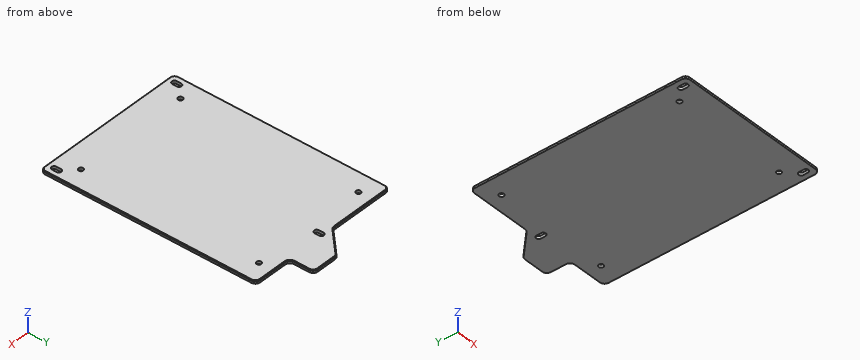
Autodesk Inventor part; units mm, degrees
ref_plane "YZ Plane" through (0, 0, 0) normal (1, 0, 0) x (0, 1, 0)
ref_plane "XZ Plane" through (0, 0, 0) normal (0, 1, 0) x (-1, 0, 0)
ref_plane "XY Plane" through (0, 0, 0) normal (0, 0, 1) x (1, 0, 0)
sketch "Sketch1" plane through (0, 0, 0) normal (0, 0, 1) x (1, 0, 0)
  line L0 (-82.5, -114.5) -> (82.5, -114.5)
  line L1 (82.5, -114.5) -> (82.5, 114.5)
  line L2 (82.5, 114.5) -> (-82.5, 114.5)
  line L3 (-82.5, 114.5) -> (-82.5, -114.5)
  line L4 (-82.5, -114.5) -> (82.5, 114.5) construction
  line L5 (82.5, -114.5) -> (-82.5, 114.5) construction
  circle A0 centre (61.5, 99.5) radius 2.5
  line L6 (-147.2223, 0) -> (154.3177, 0) construction
  line L7 (-104.1452, 5) -> (111.2405, 5) construction
  circle A1 centre (61.5, -89.5) radius 2.5
  line L8 (0, 191.5) -> (0, -165.5) construction
  circle A2 centre (-61.5, 99.5) radius 2.5
  circle A3 centre (-61.5, -89.5) radius 2.5
  line L9 (41.5, 114.5) -> (41.5, 140.5)
  line L10 (41.5, 140.5) -> (13.216, 140.5)
  line L11 (13.216, 140.5) -> (-12.784, 114.5)
  point P0 (0, 0)
  dimension "d0" = 229
  dimension "d1" = 165
  dimension "d3" = 5
  dimension "d5" = 189
  dimension "d6" = 25
  dimension "d9" = 61.5
  dimension "d31" = 41
  dimension "d32" = 26
  dimension "d33" = 135
  dimension "d34" = 28.284
extrude "Plate1" add sketch "Sketch1" along normal blind 3
fillet "Fillet1" radius 5 4 edges at (-82.5, 114.5, 1.5) (82.5, 114.5, 1.5) (82.5, -114.5, 1.5) (-82.5, -114.5, 1.5)
sketch "Sketch2" plane through (0, 0, 3) normal (0, 0, 1) x (1, 0, 0)
  line L0 (-74.3, -107) -> (-74.3, -102) construction
  line L1 (-76.95, -107) -> (-76.95, -102)
  line L2 (-71.65, -102) -> (-71.65, -107)
  arc A0 (-76.95, -107) -> (-71.65, -107) centre (-74.3, -107) ccw
  arc A1 (-71.65, -102) -> (-76.95, -102) centre (-74.3, -102) ccw
  line L3 (-103.0799, -19.5) -> (98.9164, -19.5) construction
  line L4 (0, 191.5) -> (0, -165.5) construction
  line L5 (-82.5, -109.5) -> (-82.5, 109.5) construction
  line L6 (74.3, -107) -> (74.3, -102) construction
  line L7 (76.95, -107) -> (76.95, -102)
  line L8 (71.65, -102) -> (71.65, -107)
  arc A2 (71.65, -107) -> (76.95, -107) centre (74.3, -107) ccw
  arc A3 (76.95, -102) -> (71.65, -102) centre (74.3, -102) ccw
  line L9 (77.5, -114.5) -> (-77.5, -114.5)
  line L10 (0, 113) -> (0, 108) construction
  line L11 (-2.65, 113) -> (-2.65, 108)
  line L12 (2.65, 108) -> (2.65, 113)
  arc A4 (2.65, 113) -> (-2.65, 113) centre (0, 113) ccw
  arc A5 (-2.65, 108) -> (2.65, 108) centre (0, 108) ccw
  line L13 (-77.5, 114.5) -> (77.5, 114.5)
  point P0 (0, 0)
  point P1 (-74.3, -104.5)
  point P2 (74.3, -104.5)
  point P3 (82.5, -109.5)
  point P4 (0, 110.5)
  dimension "d12" = 85
  dimension "d14" = 5
  dimension "d15" = 2.65
  dimension "d18" = 10
  dimension "d22" = 148.6
  dimension "d23" = 5
  dimension "d24" = 2.65
  dimension "d26" = 225
extrude "Cut1" cut sketch "Sketch2" against normal blind 3
fillet "Fillet2" radius 5 4 edges at (41.5, 114.5, 1.5) (41.5, 140.5, 1.5) (13.216, 140.5, 1.5) (-12.784, 114.5, 1.5)
chamfer "Chamfer1" distance 0.75 angle 45 14 edges at (0, -114.5, 3) (-81.0355, -113.0355, 3) (-82.5, 0, 3) (-81.0355, 113.0355, 3) (-46.1775, 114.5, 3) (13.3737, 140.1194, 3) (40.0355, 139.0355, 3) (0.216, 127.5, 3) (25.8935, 140.5, 3) (41.5, 127.5, 3) (62, 114.5, 3) (81.0355, 113.0355, 3) (82.5, 0, 3) (81.0355, -113.0355, 3)
sketch "Sketch4" plane through (0, 0, 3) normal (0, 0, 1) x (1, 0, 0)
  circle A0 centre (85, -108.7631) radius 2
  line L0 (82.5, -109.5) -> (82.5, 109.5)
  point P0 (0, 0)
  dimension "d35" = 2.5
  dimension "d36" = 4
equation "\"d3\" = d2"
equation "\"d15\" = d24"
equation "\"d23\" = d14"
equation "\"d16\" = Thickness"
equation "\"d10\" = Thickness"
equation "\"BendRadius\" = Thickness"
equation "\"BendReliefWidth\" = Thickness"
equation "\"BendReliefDepth\" = 0.5 * Thickness"
equation "\"CornerReliefSize\" = 4 * Thickness"
equation "\"MinimumRemnant\" = 2 * Thickness"
equation "\"TransitionRadius\" = BendRadius"
equation "\"JacobiRadiusSize\" = BendRadius"
equation "\"GapSize\" = Thickness"
properties part number "TBD_Box_Fix"
Geometry check sheet. Reference: the model listing, model coordinates, mm. Round coordinates to 2 decimals unless told otherwise and drop trailing zeros. Loops run counter-clockwise (first coordinate to the right, second up) from the corner with the lowest first, then second, coordinate; pieces in that order, holes last. Notation, with made-up numbers: (43, 66.5) -> (51, 66.5) arc R27 cw to (51, 89.5) -> close; hole circle Ø9 at (-34, 83). An arc over 180 degrees is marked (long way). Answer as a JSON object with one key per item and string values. Group by question number.
Item 1: Cross-section at B-B, the plane z = 1.25. Count the separate pieces of the cut face and the enclosed holes in it, plus the area to 3 significant figures.
Item 2: Thickness scan on line 1 along Y through (x, z) = (61.5, 1.15); line 2 along Y through (x, z) = (-61.5, 2.3); line 3 along Y through (x, z) = (53.5, 2.15). Record the ranges inside material, lowest first.
Item 3: Cross-section at D-D, the plane x = -32. Record the cut outline in (y, z).
Item 4: Cross-section at A-A, the plane x = 61.5. Record the cut outline in (y, z).
Item 5: Cross-section at C-C, the plane x = 0. Record the cut outline in (y, z).
Item 6: Depth check by flat-ended pin: pin 1 Ø0.7 at (y, z) = (131, 1.5) entering from +X; pin 2 Ø1 at (x, z) = (44, 1) entering from +Y; pin 3 Ø1 at (x, z) = (-53, 2) entering from +Y. Enter the tip coordinate at first touch or a pass-through.
Determined:
{
 "1": {"separate pieces": "1", "enclosed holes": "7", "area": "38,600 mm²"},
 "2": {"line 1": "y = -114.5 to -92, -87 to 97, 102 to 114.5", "line 2": "y = -114.45 to -92, -87 to 97, 102 to 114.45", "line 3": "y = -114.5 to 114.5"},
 "3": {"outline": "(-114.5, 0) -> (114.5, 0) -> (114.5, 2.25) -> (113.75, 3) -> (-113.75, 3) -> (-114.5, 2.25) -> close"},
 "4": {"outline": "(-114.5, 0) -> (-92, 0) -> (-92, 3) -> (-113.75, 3) -> (-114.5, 2.25) -> close; (-87, 0) -> (97, 0) -> (97, 3) -> (-87, 3) -> close; (102, 0) -> (114.5, 0) -> (114.5, 2.25) -> (113.75, 3) -> (102, 3) -> close"},
 "5": {"outline": "(-114.5, 0) -> (105.35, 0) -> (105.35, 3) -> (-113.75, 3) -> (-114.5, 2.25) -> close; (115.65, 0) -> (127.28, 0) -> (127.28, 2.25) -> (126.22, 3) -> (115.65, 3) -> close"},
 "6": {"pin 1": "stops at x = 41.5", "pin 2": "stops at y = 115.5", "pin 3": "stops at y = 114.5"}
}
